from build123d import *

# Parameters (mm, degrees)
BOSS_EXTRUDE1_DEPTH      = 0.0001
BOSS_EXTRUDE1_DEPTH_BACK = 248
BOSS_EXTRUDE2_DEPTH      = 25
CUT_EXTRUDE1_DEPTH       = 20
BOSS_EXTRUDE3_DEPTH      = 25
CUT_EXTRUDE2_DEPTH       = 20
BOSS_EXTRUDE4_DEPTH      = 5
BOSS_EXTRUDE5_DEPTH      = 5
SKETCH8_R                = 1.5
CUT_EXTRUDE3_DEPTH       = 10
SKETCH9_W                = 70
SKETCH9_H                = 5.120472302
BOSS_EXTRUDE7_DEPTH      = 250
SKETCH11_W               = 70
SKETCH11_H               = 5.120472302
CUT_EXTRUDE4_DEPTH       = 250
CUT_EXTRUDE5_DEPTH       = 2


with BuildPart() as part:
    # Sketch1 → Boss-Extrude1 (new, two sides: drawn at the far end of the back side and taken through both)
    with BuildSketch(Plane(origin=(0, 0, 0), x_dir=(0, 0, -1), z_dir=(1, 0, 0)).offset(-BOSS_EXTRUDE1_DEPTH_BACK)):
        Polygon((-23.04212536, -5.120472302), (67.5, 35.120472302), (158.04212536, -5.120472302), (158.04212536, -10.240944604), (135, 0), (67.5, 30), (0, 0), (-23.04212536, -10.240944604), align=None)
    extrude(amount=BOSS_EXTRUDE1_DEPTH + BOSS_EXTRUDE1_DEPTH_BACK)

    # Sketch2 → Boss-Extrude2 (add)
    with BuildSketch(Plane(origin=(0.0001, 0, 0), x_dir=(0, 0, -1), z_dir=(1, 0, 0))):
        Polygon((0, 0), (135, 0), (67.5, 30), align=None)
    extrude(amount=-BOSS_EXTRUDE2_DEPTH)

    # Sketch3 → Cut-Extrude1 (cut)
    with BuildSketch(Plane(origin=(0.0001, 0, 0), x_dir=(0, 0, -1), z_dir=(1, 0, 0))):
        Polygon((0, 0), (135, 0), (67.5, 30), align=None)
    extrude(amount=-CUT_EXTRUDE1_DEPTH, mode=Mode.SUBTRACT)

    # Sketch4 → Boss-Extrude3 (add)
    with BuildSketch(Plane.ZY.offset(248)):
        Polygon((-135, 0), (0, 0), (-67.5, 30), align=None)
    extrude(amount=-BOSS_EXTRUDE3_DEPTH)

    # Sketch5 → Cut-Extrude2 (cut)
    with BuildSketch(Plane.ZY.offset(248)):
        Polygon((-135, 0), (0, 0), (-67.5, 29.582678365), align=None)
    extrude(amount=-CUT_EXTRUDE2_DEPTH, mode=Mode.SUBTRACT)

    # Sketch6 → Boss-Extrude4 (add)
    with BuildSketch(Plane(origin=(0, 0, 0), x_dir=(-1, 0, 0), z_dir=(0, -1, 0))):
        with BuildLine():
            ThreePointArc((233.3, 67.5), (235, 69.2), (236.7, 67.5))
            Line((236.7, 67.5), (242, 67.5))
            ThreePointArc((242, 67.5), (237.899494937, 77.399494937), (228, 81.5))
            Line((228, 81.5), (228, 67.5))
            Line((228, 67.5), (233.3, 67.5))
        make_face()
        with BuildLine():
            Line((242, 67.5), (236.7, 67.5))
            ThreePointArc((236.7, 67.5), (235, 65.8), (233.3, 67.5))
            Line((233.3, 67.5), (228, 67.5))
            Line((228, 67.5), (228, 53.5))
            ThreePointArc((228, 53.5), (237.899494937, 57.600505063), (242, 67.5))
        make_face()
        with BuildLine():
            Line((223, 54.423303169), (223, 80.576696831))
            ThreePointArc((223, 80.576696831), (214, 67.5), (223, 54.423303169))
        make_face()
        with BuildLine():
            Line((228, 67.5), (228, 81.5))
            ThreePointArc((228, 81.5), (225.457732865, 81.267239295), (223, 80.576696831))
            Line((223, 80.576696831), (223, 54.423303169))
            ThreePointArc((223, 54.423303169), (225.457732865, 53.732760705), (228, 53.5))
            Line((228, 53.5), (228, 67.5))
        make_face()
    extrude(amount=-BOSS_EXTRUDE4_DEPTH)

    # Sketch7 → Boss-Extrude5 (add)
    with BuildSketch(Plane(origin=(0, 0, 0), x_dir=(-1, 0, 0), z_dir=(0, -1, 0))):
        with BuildLine():
            Line((19.9999, 57.5001), (19.9999, 67.5))
            Line((19.9999, 67.5), (16.69995, 67.5))
            ThreePointArc((16.69995, 67.5), (14.99995, 65.8), (13.29995, 67.5))
            Line((13.29995, 67.5), (10, 67.5))
            ThreePointArc((10, 67.5), (12.928902899, 60.429002899), (19.9999, 57.5001))
        make_face()
        with BuildLine():
            Line((16.69995, 67.5), (19.9999, 67.5))
            Line((19.9999, 67.5), (19.9999, 77.4999))
            ThreePointArc((19.9999, 77.4999), (12.928902899, 74.570997101), (10, 67.5))
            Line((10, 67.5), (13.29995, 67.5))
            ThreePointArc((13.29995, 67.5), (14.99995, 69.2), (16.69995, 67.5))
        make_face()
        with BuildLine():
            Line((19.9999, 77.4999), (19.9999, 67.5))
            Line((19.9999, 67.5), (19.9999, 57.5001))
            ThreePointArc((19.9999, 57.5001), (22.588092453, 57.840845801), (24.9999, 58.839861432))
            Line((24.9999, 58.839861432), (24.9999, 76.160138568))
            ThreePointArc((24.9999, 76.160138568), (22.588092453, 77.159154199), (19.9999, 77.4999))
        make_face()
        with BuildLine():
            ThreePointArc((29.9998, 67.5), (28.660081869, 72.499925), (24.9999, 76.160138568))
            Line((24.9999, 76.160138568), (24.9999, 58.839861432))
            ThreePointArc((24.9999, 58.839861432), (28.660081869, 62.500075), (29.9998, 67.5))
        make_face()
    extrude(amount=-BOSS_EXTRUDE5_DEPTH)

    # Sketch8 → Cut-Extrude3 (cut)
    with BuildSketch(Plane.ZY.offset(228)):
        with Locations((-67.5, 25)):
            Circle(SKETCH8_R)
    extrude(amount=-CUT_EXTRUDE3_DEPTH, mode=Mode.SUBTRACT)

    # Sketch9 → Boss-Extrude7 (add)
    with BuildSketch(Plane.ZY.offset(248)):
        with Locations((58.04212536, -7.680708453)):
            Rectangle(SKETCH9_W, SKETCH9_H)
    extrude(amount=-BOSS_EXTRUDE7_DEPTH)

    # Sketch11 → Cut-Extrude4 (cut)
    with BuildSketch(Plane.ZY.offset(248)):
        with Locations((58.04212536, -7.680708453)):
            Rectangle(SKETCH11_W, SKETCH11_H)
    extrude(amount=-CUT_EXTRUDE4_DEPTH, mode=Mode.SUBTRACT)

    # Sketch12 → Cut-Extrude5 (cut)
    with BuildSketch(Plane(origin=(0.0001, 0, 0), x_dir=(0, 0, -1), z_dir=(1, 0, 0))):
        Polygon((-23.04212536, -5.120472302), (67.5, 35.120472302), (158.04212536, -5.120472302), (158.04212536, -10.240944604), (67.5, 30), (-23.04212536, -10.240944604), align=None)
    extrude(amount=-CUT_EXTRUDE5_DEPTH, mode=Mode.SUBTRACT)


solid = part.part
Source: CAD feature listing. Evaluate the final solid. Frame: model axes, mm. A direction names the side the tool comes from. Round coordinates to 2 decimals unless told otherwise and drop trailing zeros. Loops run counter-clockwise (first coordinate to the right, second up) from the corner with the lowest first, then second, coordinate; pieces in that order, holes last. Notation, with made-up numbers: (-29.75, 47.25) -> (26.25, 47.25) arc R21 cw to (26.25, 52.25) -> close; hole circle Ø10 at (27.25, 10). An arc over 180 degrees is marked (long way). Answer as a JSON object with one key per item and string values. Group by question number.
Q1. Ray query, line 1 (X direction, y = 1.1, z = -67.5); line 2 (X direction, y = 8.5, z = -31); line 3 (Z direction, x = -235, y = 2). Return the intervals inside material, ascending. Write a range as from..to.
Q2. Contact query for flat-ended pins moving along their axis: P1, Ø4, axis at x = -36.5, y = 18.5, coming from the +Z side; P2, Ø6, axis at x = -109.5, z = -50, coming from the +Y side; P3, Ø3.5, axis at y = 25, z = -67.5, coming from the -X side. Output: stop coordinate, or through.
Q3. Mould query, pull axis X, two halves, no side actions, for faces 1 (the flat face through (-228, 8, -68)), 2 (the flat face through (-2, 28, -75)), 3 (the flat face through (-20, 0, -68)), 4 (the cylindrical face through (-214, 2.5, -67.7)). Classes: pulls with the +X half, pulls with the -X half, needs draft (parallel to the pull), parting line crosses it, or undercut.
Q4. Section query C-C (z = -29). Output: boundary loops of the cut face in (x, y).
Q5. Section query B-B (z = -127). Output: boundary loops of the cut face in (x, y), plus the area to 3 significant figures.
Q6. Section query A-A (x = -118.5). Output: boundary loops of the cut face in (y, z), plus the area to 3 significant figures.
Q7. Access query for faces 5 (the flat face through (-25, 12, -67)), 6 (the flat face through (-232, 5, -68)), 7 (the flat face through (-227, 0, -68)). Directions: +Z, -Z, +X, -X, +Y, -Y. A direction counts if a zero-diameter tool reaches every point of the face in a straight line with its end or side. Return the directions, or none.
Completed:
{
 "1": {"line 1": "-242..-236.7, -233.3..-214, -30..-16.7, -13.3..-10", "line 2": "-228..-223, -25..-20", "line 3": "-142.02..-130.44, -79.62..-69.2, -65.8..-55.38, -4.56..7.02"},
 "2": {"P1": "z = -25.6", "P2": "y = 28.68", "P3": "x = -228"},
 "3": {"face 1": "pulls with the -X half", "face 2": "pulls with the +X half", "face 3": "needs draft", "face 4": "undercut"},
 "4": {"outline": "(-248, 12.71) -> (-228, 12.71) -> (-228, 0) -> (-223, 0) -> (-223, 12.89) -> (-25, 12.89) -> (-25, 0) -> (-20, 0) -> (-20, 12.89) -> (-2, 12.89) -> (-2, 18.01) -> (-248, 18.01) -> close"},
 "5": {"outline": "(-248, 3.51) -> (-228, 3.51) -> (-228, 0) -> (-223, 0) -> (-223, 3.56) -> (-25, 3.56) -> (-25, 0) -> (-20, 0) -> (-20, 3.56) -> (-2, 3.56) -> (-2, 8.68) -> (-248, 8.68) -> close", "area": "1,300 mm²"},
 "6": {"outline": "(-10.24, -158.04) -> (-5.12, -158.04) -> (35.12, -67.5) -> (-5.12, 23.04) -> (-10.24, 23.04) -> (30, -67.5) -> close", "area": "927 mm²"},
 "7": {"face 5": "none", "face 6": "-X", "face 7": "+X, -X, -Y"}
}
